Source: CAD feature listing. Evaluate the final solid. Frame: model axes, mm. Face numbers are marked on the shaded views. A direction names the side the tool comes from. Give positions to 0.01 mm unless a question says otherwise; leave off trailing zeros. Order: outer loops, then holes, each group sorted by start corner. A loop starts at its lowest first (then second) coordinate and runs counter-clockwise, first axis right, second up.
1) Section C-C, the plane y = 23.5. Return loops of the section in (x, z), plus the area to 3 significant figures.
2) Access query for the marked faces 1 and 2. Directions: +Z, -Z, +X, -X, +Y, -Y. A direction counts if a zero-diameter tool reaches every point of the face in a straight line with its end or side. Return the directions, or none.
3) Section B-B, the plane z = 34. Return loops of the section in (x, y), plus the area to 3 significant figures.
4) First-contact query: P1, Ø10, axis at x = 21, y = 55.5, coming from the +Z side. Flat tip, straight axial feed; report the tip coordinate or a pass-through.
5) Section A-A, the plane z = 22. Return loops of the section in (x, y).
6) Section D-D, the plane y = -31. Return loops of the section in (x, z), plus the area to 3 significant figures.
7) Material intervals for line 1 (Y direction, x = 49.75, z = 22); line 2 (X direction, y = -20.5, z = 35.5); line 3 (X direction, y = 78.5, z = 0.5), sorted ascending.
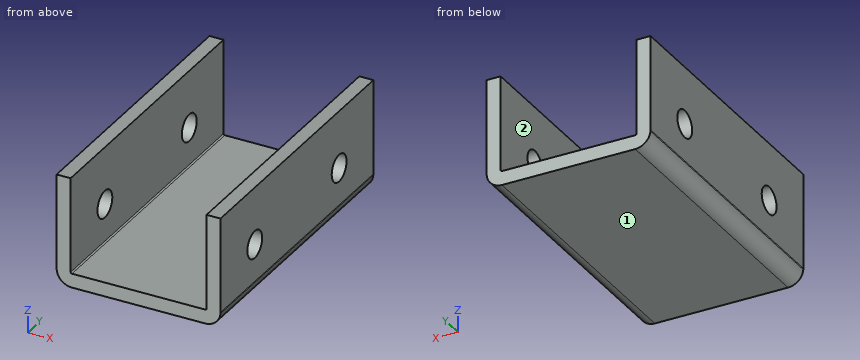
```python
from build123d import *

# Parameters (mm, degrees)
CROQUIS1_W                    = 199
CROQUIS1_H                    = 160
BRIDA_BASE1_DEPTH             = 8
PLIEGUE_START                 = -62.828947368
PLIEGUE_CROQUIZADO1_DEPTH     = 160
PLIEGUE_CROQUIZADO1_2_DEPTH   = 160
TALADRO_DE_MARGEN_PARA_M141_D = 15.5


# Read off the part's stored shape, not the designer's step: Pliegue croquizado1
# Sheet-metal steps are written as plain solids
with BuildPart() as part:
    # Croquis1 → Brida base1 (new body)
    with BuildSketch(Plane.XY):
        with Locations((8.132704294, 17.171052632)):
            Rectangle(CROQUIS1_W, CROQUIS1_H)
    extrude(amount=-BRIDA_BASE1_DEPTH)

    # Pliegue croquizado1 outline → Pliegue croquizado1 (cut)
    with BuildSketch(Plane(origin=(0, 0, 0), x_dir=(1, 0, 0), z_dir=(0, 1, 0)).offset(PLIEGUE_START)):
        with BuildLine():
            Line((107.632704294, 8), (46.146104294, 8))
            ThreePointArc((46.146104294, 8), (52.057652315, 5.696267134), (54.851596813, 0))
            Line((54.851596813, 0), (107.632704294, 0))
            Line((107.632704294, 0), (107.632704294, 8))
        make_face()
        with BuildLine():
            ThreePointArc((-38.586188225, 0), (-35.792243727, 5.696267134), (-29.880695706, 8))
            Line((-29.880695706, 8), (-91.367295706, 8))
            Line((-91.367295706, 8), (-91.367295706, 0))
            Line((-91.367295706, 0), (-38.586188225, 0))
        make_face()
    extrude(amount=PLIEGUE_CROQUIZADO1_DEPTH, mode=Mode.SUBTRACT)

    # Pliegue croquizado1 2 outline → Pliegue croquizado1 2 (add)
    with BuildSketch(Plane(origin=(0, 0, 0), x_dir=(1, 0, 0), z_dir=(0, 1, 0)).offset(PLIEGUE_START)):
        with BuildLine():
            ThreePointArc((54.882704294, -0.7366), (54.874923959, -0.36797172), (54.851596813, 0))
            Line((54.851596813, 0), (46.146104294, 0))
            ThreePointArc((46.146104294, 0), (46.666959149, -0.215745145), (46.882704294, -0.7366))
            Line((46.882704294, -0.7366), (46.882704294, -54.782966119))
            Line((46.882704294, -54.782966119), (54.882704294, -54.782966119))
            Line((54.882704294, -54.782966119), (54.882704294, -0.7366))
        make_face()
        with BuildLine():
            Line((-29.880695706, 0), (-38.586188225, 0))
            ThreePointArc((-38.586188225, 0), (-38.609515371, -0.36797172), (-38.617295706, -0.7366))
            Line((-38.617295706, -0.7366), (-38.617295706, -54.782966119))
            Line((-38.617295706, -54.782966119), (-30.617295706, -54.782966119))
            Line((-30.617295706, -54.782966119), (-30.617295706, -0.7366))
            ThreePointArc((-30.617295706, -0.7366), (-30.401550561, -0.215745145), (-29.880695706, 0))
        make_face()
    extrude(amount=PLIEGUE_CROQUIZADO1_2_DEPTH)

    # Taladro de margen para M141 (through all)
    with Locations(Plane.ZY.offset(38.617295706)):
        with Locations((22, -26.978947368), (22, 61.321052632)):
            Hole(TALADRO_DE_MARGEN_PARA_M141_D / 2)


solid = part.part
```
From the geometry:
1. outline: (-38.62, 0.74) arc R8.74 ccw to (-29.88, -8) - (46.15, -8) arc R8.74 ccw to (54.88, 0.74) - (54.88, 54.78) - (46.88, 54.78) - (46.88, 0.74) arc R0.74 cw to (46.15, 0) - (-29.88, 0) arc R0.74 cw to (-30.62, 0.74) - (-30.62, 54.78) - (-38.62, 54.78) - close
1. area: 1,590 mm2
2. face 1: -Z, +X, -X, +Y, -Y
2. face 2: +Z, +Y, -Y
3. outline: (-38.62, -62.83) - (-30.62, -62.83) - (-30.62, 97.17) - (-38.62, 97.17) - close; (46.88, -62.83) - (54.88, -62.83) - (54.88, 97.17) - (46.88, 97.17) - close
3. area: 2,560 mm2
4. P1: stops at z = 0
5. outline: (-38.62, -62.83) - (-30.62, -62.83) - (-30.62, -34.73) - (-38.62, -34.73) - close; (-38.62, -19.23) - (-30.62, -19.23) - (-30.62, 53.57) - (-38.62, 53.57) - close; (-38.62, 69.07) - (-30.62, 69.07) - (-30.62, 97.17) - (-38.62, 97.17) - close; (46.88, -62.83) - (54.88, -62.83) - (54.88, -34.73) - (46.88, -34.73) - close; (46.88, -19.23) - (54.88, -19.23) - (54.88, 53.57) - (46.88, 53.57) - close; (46.88, 69.07) - (54.88, 69.07) - (54.88, 97.17) - (46.88, 97.17) - close
6. outline: (-38.62, 0.74) arc R8.74 ccw to (-29.88, -8) - (46.15, -8) arc R8.74 ccw to (54.88, 0.74) - (54.88, 15.37) - (46.88, 15.37) - (46.88, 0.74) arc R0.74 cw to (46.15, 0) - (-29.88, 0) arc R0.74 cw to (-30.62, 0.74) - (-30.62, 15.37) - (-38.62, 15.37) - close; (-38.62, 28.63) - (-30.62, 28.63) - (-30.62, 54.78) - (-38.62, 54.78) - close; (46.88, 28.63) - (54.88, 28.63) - (54.88, 54.78) - (46.88, 54.78) - close
6. area: 1,380 mm2
7. line 1: y = -62.83 to -34.73, -19.23 to 53.57, 69.07 to 97.17
7. line 2: x = -38.62 to -30.62, 46.88 to 54.88
7. line 3: x = -38.61 to -30.58, 46.84 to 54.88
